The drawing under review shows one solid part. Ordinate dimensions are in mm from its lowest x, y, z. A direction names the side the tool comes from. Coordinates: 2 decimals unless noted, no trailing zeros. Order: outer loops, then holes, each group sorted by start corner. A loop starts at its lowest first (then second) coordinate and runs counter-clockwise, first axis right, second up. Notation, with made-up numbers: (48.5, 2) -> (70.5, 2) arc R14 cw to (70.5, 17) -> close; hole circle Ø11 at (-21, 49.25). An arc over 180 degrees is marked (long way). Put each result on its own line as item: value.
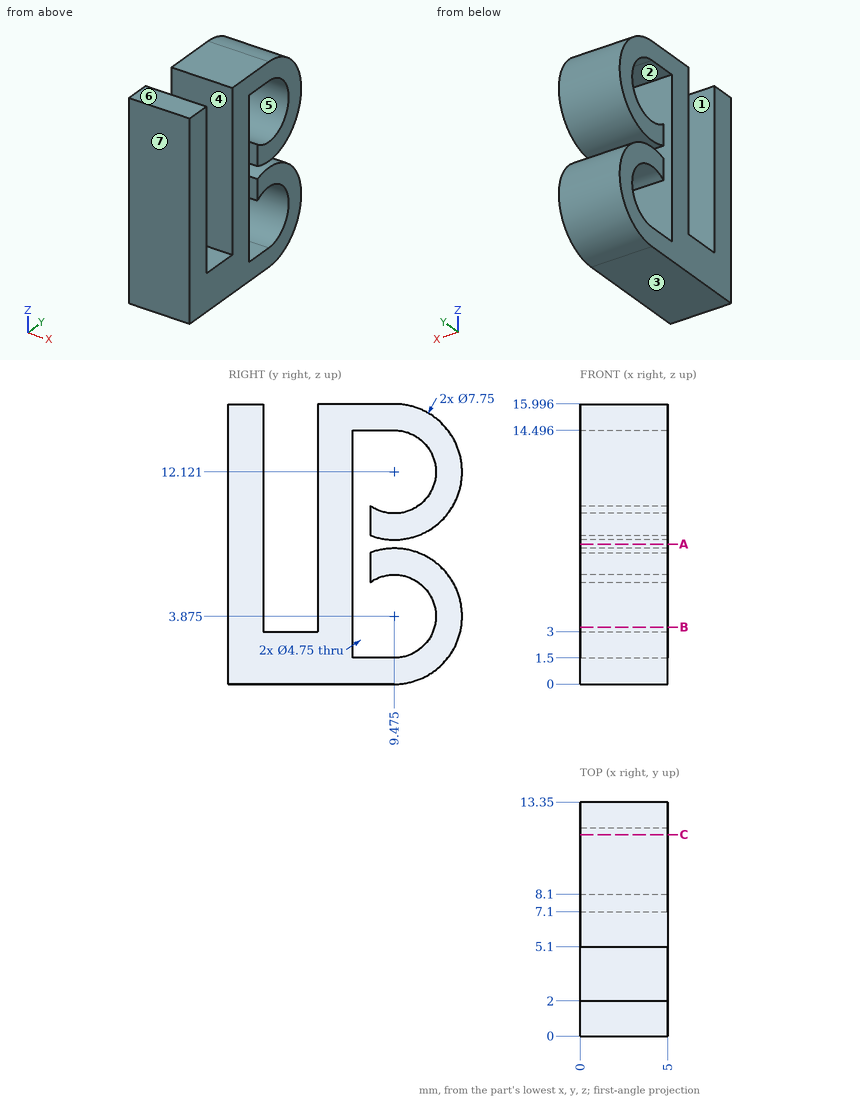
Item 1: Consider section B-B on z = 3.25. Write out the cut boundary in (x, y).
Answers below:
outline: (0, 0) -> (5, 0) -> (5, 2) -> (0, 2) -> close; (0, 5.1) -> (5, 5.1) -> (5, 7.1) -> (0, 7.1) -> close; (0, 11.77) -> (5, 11.77) -> (5, 13.3) -> (0, 13.3) -> close
Item 2: Consider section A-A on z = 8. Write out the cut boundary in (x, y), and give its area (3 significant figures).
Answers below:
outline: (0, 0) -> (5, 0) -> (5, 2) -> (0, 2) -> close; (0, 5.1) -> (5, 5.1) -> (5, 7.1) -> (0, 7.1) -> close
area: 20.0 mm^2
Item 3: For the marked faces 1, 2 and 3, list the 3-axis set-ups (+Z, -Z, +X, -X, +Y, -Y) from which the entire face can be reached by the end or side of a thin tool; tool diameter is ignored.
Answers below:
face 1: +Z, +X, -X
face 2: +X, -X
face 3: -Z, +X, -X, +Y, -Y
Item 4: For line 1 (Z direction, x = 0.95, y = 7.25); line 2 (Y direction, x = 3.85, z = 14) (1 decimal); line 3 (Z direction, x = 2.35, y = 9.25) (1 decimal), list the stretches that pass through material, from the lowest coordinate up. Write a range as from..to.
Answers below:
line 1: 0..1.5, 14.5..16
line 2: 0..2, 5.1..7.1, 10.9..12.9
line 3: 0..1.5, 6.2..7.7, 8.3..9.8, 14.5..16
Item 5: Consider section C-C on y = 11.5. Write out the cut boundary in (x, z) (1 decimal).
Answers below:
outline: (0, 0.6) -> (5, 0.6) -> (5, 2.6) -> (0, 2.6) -> close; (0, 5.1) -> (5, 5.1) -> (5, 7.2) -> (0, 7.2) -> close; (0, 8.8) -> (5, 8.8) -> (5, 10.9) -> (0, 10.9) -> close; (0, 13.4) -> (5, 13.4) -> (5, 15.4) -> (0, 15.4) -> close
Item 6: Mouldability with a two-part tool opening along Y and no side actions: class the marked faces 4, 5, 6 and 7 as +Y half, -Y half, draft (parallel to the pull), parting line (faces both ways), or undercut.
Answers below:
face 4: undercut
face 5: undercut
face 6: draft
face 7: -Y half
Item 7: For pin 1 Ø1.5 at (x, z) = (4.5, 6.5) entering from +Y; pin 2 Ø1.5 at (x, z) = (3.5, 8.5) entering from +Y; pin 3 Ø2.5 at (x, z) = (3, 6.5) entering from +Y; pin 4 Ø4 at (y, z) = (9.475, 3.875) entering from +X, all flat-tipped, find the tip position at first contact; note any pin that passes through.
Answers below:
pin 1: y = 12.87
pin 2: y = 12.08
pin 3: y = 13.1
pin 4: through
